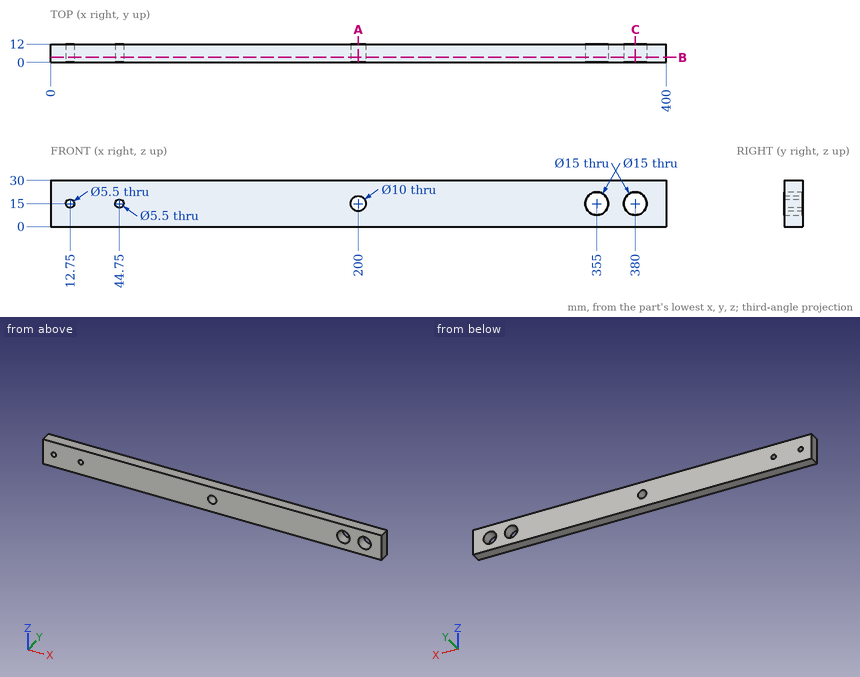
Design review of the part shown in the three views and the two pictorial views. Dimensions are in mm from the part's minimum x, y and z. Give positions to 0.01 mm unless a question says otherwise; leave off trailing zeros. Write each loop counter-clockwise with the first axis right and the second up, starting at its lowest first coordinate (ties: lowest second). Pieces come first, ordered by that corner, then holes. Notation, with made-up numbers: M -32,0.5 L 27,0.5 A8 ccw 27,7.5 Z; hole C -37.75,24.5 d6. An arc over 180 degrees is marked long. One line per question, with ' | ' between items. Start each with the question number.
Item 1: For pin 1 (6.5 mm diameter, centred on x = 44.75, z = 15, fed in from -Y); pin 2 (12 mm diameter, centred on x = 380, z = 15, fed in from -Y), all flat-tipped, find the tip position at first contact; note any pin that passes through.
Item 2: We need section A-A on x = 200. Write out the cut boundary in (y, z).
Item 3: Wall thickness on line 1 (X direction, y = 8.25, z = 15); line 2 (Z direction, x = 12.75, y = 6); line 3 (Z direction, x = 380, y = 5.75): over which ranges is each line inside the solid? List them lowest first. Write a range as from..to.
Item 4: We need section C-C on x = 380. Write out the cut boundary in (y, z).
Item 5: We need section B-B on y = 3.25. Write out the cut boundary in (x, z), plus the area to 3 significant figures.
Results found:
1) pin 1: stops at y = 0 | pin 2: passes through
2) outline: M 0,0 L 12,0 L 12,10 L 0,10 Z; M 0,20 L 12,20 L 12,30 L 0,30 Z
3) line 1: x = 0..10, 15.5..42, 47.5..195, 205..347.5, 362.5..372.5, 387.5..400 | line 2: z = 0..12.25, 17.75..30 | line 3: z = 0..7.5, 22.5..30
4) outline: M 0,0 L 12,0 L 12,7.5 L 0,7.5 Z; M 0,22.5 L 12,22.5 L 12,30 L 0,30 Z
5) outline: M 0,0 L 400,0 L 400,30 L 0,30 Z; hole C 12.75,15 d5.5; hole C 44.75,15 d5.5; hole C 200,15 d10; hole C 355,15 d15; hole C 380,15 d15 | area: 11,500 mm2
